Input: dimensioned drawing with shaded views. Units: mm. Origin: part minimum x, y, z. A direction names the side the tool comes from. Round coordinates to 2 decimals unless told otherwise and drop trailing zeros. Write each loop counter-clockwise with the first axis right and the second up, starting at its lowest first coordinate (ties: lowest second). Pieces come first, ordered by that corner, then holes. Notation, with made-up numbers: M 20,-31 L 60,-31 A24 ccw 60,-14 Z; hole C -34.5,-32.5 d4. An arc over 180 degrees is marked long. Put each result on its own line as item: value. Start each with the question number.
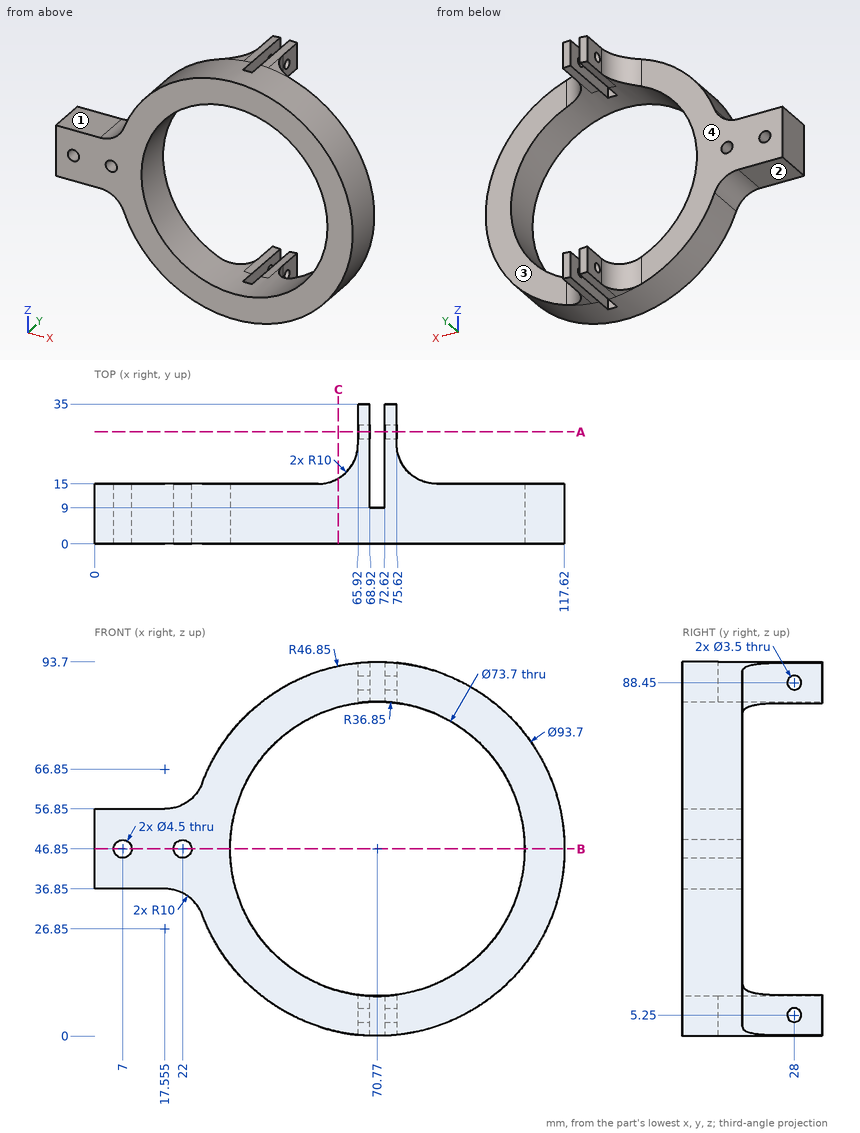
1) First-contact query: pin 1 (4.5 mm diameter, centred on x = 11.5, y = 8.5, fed in from +Z); pin 2 (11 mm diameter, centred on y = 16, z = 4.5, fed in from +X) (1 decimal); pin 3 (3 mm diameter, centred on x = 63, y = 4, fed in from -Z); pin 4 (3 mm diameter, centred on y = 28, z = 88.45, fed in from +X). Flat tips, straight axial feed; report the tip coordinate or a pass-through.
2) Access query for the marked faces 1, 2, 3 and 4. Directions: +Z, -Z, +X, -X, +Y, -Y. A direction counts if a zero-diameter tool reaches every point of the face in a straight line with its end or side. Return the directions, or none.
3) Section C-C, the plane x = 61. Output: boundary loops of the cut face in (y, z).
4) Section A-A, the plane y = 28. Give the number of separate pieces and of enclosed holes in the cut face.
5) Section B-B, the plane z = 46.85. Output: boundary loops of the cut face in (x, y).
6) Ray query, probe 1 along X at (y, z) = (14, 46.5); probe 2 along Y at (x, z) = (73.2, 5.25); probe 3 along X at (y, z) = (13, 46) (1 decimal). Return the intervals inside material, ascending.
Solved:
1. pin 1: stops at z = 56.85
1. pin 2: stops at x = 99.6
1. pin 3: stops at z = 0.42
1. pin 4: passes through
2. face 1: +Z, -X, +Y, -Y
2. face 2: -Z, -X, +Y, -Y
2. face 3: +Z, -Z, +X, +Y
2. face 4: +Z, -Z, -X, +Y
3. outline: M 0,1.03 L 16.39,1.03 L 16.39,11.32 L 0,11.32 Z; M 0,82.38 L 16.39,82.38 L 16.39,92.67 L 0,92.67 Z
4. separate pieces: 8
4. enclosed holes: 0
5. outline: M 0,0 L 4.75,0 L 4.75,15 L 0,15 Z; M 9.25,0 L 19.75,0 L 19.75,15 L 9.25,15 Z; M 24.25,0 L 33.92,0 L 33.92,15 L 24.25,15 Z; M 107.62,0 L 117.62,0 L 117.62,15 L 107.62,15 Z
6. probe 1: x = 0 to 4.78, 9.22 to 19.78, 24.22 to 33.92, 107.62 to 117.62
6. probe 2: y = 0 to 26.25, 29.75 to 35
6. probe 3: x = 0 to 4.9, 9.1 to 19.9, 24.1 to 33.9, 107.6 to 117.6
